The listing builds one solid part. Answer for the finished solid, in the listing's coordinates (mm). Round coordinates to 2 decimals unless told otherwise and drop trailing zeros. Write each loop counter-clockwise with the first axis right and the second up, starting at its lowest first coordinate (ties: lowest second). Pieces come first, ordered by that corner, then holes. Notation, with made-up numbers: (11.5, -38.5) - (49.5, -38.5) arc R6 cw to (49.5, -28.5) - close; hole circle Ø5 at (55.5, -10). An arc over 180 degrees is marked (long way). Use a Markdown table: item, result. Add a question column.
1) Find the intervals of material crossed by probe 1 along Z at (x, y) = (3.75, 444.5); probe 2 along Z at (x, y) = (1.25, 651); probe 3 along Y at (x, z) = (3.5, -644.5), in increasing order. Write a range as from..to.
2) A cutting plane is placed at A-A (x = 3). Give the vertices of the cut face in (y, z) (3 decimals), then the cut area to 3 significant figures.
3) A cutting plane is placed at B-B (z = -222). Give the vertices of the cut face in (x, y).
4) This flat-tipped pin is pushed along its axis until it touches: P1, Ø1.9, axis at x = 4.5, z = -584, coming from the +Y side. Where does it stop, or does it pass through?
```python
from build123d import *

# Parameters (mm, degrees)
SKETCH1_R           = 2.45745
BOSS_EXTRUDE1_DEPTH = 6.35


with BuildPart() as part:
    # Sketch1 → Boss-Extrude1 (new body)
    with BuildSketch(Plane(origin=(0, 0, 0), x_dir=(0, 0, -1), z_dir=(1, 0, 0))):
        with BuildLine():
            Line((457.2, 546.1), (755.65, 546.1))
            ThreePointArc((755.65, 546.1), (760.140128061, 544.240128061), (762, 539.75))
            Line((762, 539.75), (762, 6.35))
            ThreePointArc((762, 6.35), (760.140128061, 1.859871939), (755.65, 0))
            Line((755.65, 0), (6.35, 0))
            ThreePointArc((6.35, 0), (1.859871939, 1.859871939), (0, 6.35))
            Line((0, 6.35), (0, 539.75))
            ThreePointArc((0, 539.75), (1.859871939, 544.240128061), (6.35, 546.1))
            Line((6.35, 546.1), (304.8, 546.1))
            ThreePointArc((304.8, 546.1), (313.780256121, 549.819743879), (317.5, 558.8))
            Line((317.5, 558.8), (317.5, 685.8))
            ThreePointArc((317.5, 685.8), (321.219743879, 694.780256121), (330.2, 698.5))
            Line((330.2, 698.5), (431.8, 698.5))
            ThreePointArc((431.8, 698.5), (440.780256121, 694.780256121), (444.5, 685.8))
            Line((444.5, 685.8), (444.5, 558.8))
            ThreePointArc((444.5, 558.8), (448.219743879, 549.819743879), (457.2, 546.1))
        make_face()
        with Locations((53.975, 444.5)):
            Circle(SKETCH1_R, mode=Mode.SUBTRACT)
        with Locations((708.025, 444.5)):
            Circle(SKETCH1_R, mode=Mode.SUBTRACT)
        with Locations((708.025, 238.125)):
            Circle(SKETCH1_R, mode=Mode.SUBTRACT)
        with Locations((53.975, 238.125)):
            Circle(SKETCH1_R, mode=Mode.SUBTRACT)
        with Locations((53.975, 187.325)):
            Circle(SKETCH1_R, mode=Mode.SUBTRACT)
        with Locations((708.025, 187.325)):
            Circle(SKETCH1_R, mode=Mode.SUBTRACT)
    extrude(amount=BOSS_EXTRUDE1_DEPTH)


solid = part.part
```
Entries:
| question | item | result |
|---|---|---|
| 1 | probe 1 | z = -762..-710.48, -705.57..-56.43, -51.52..0 |
| 1 | probe 2 | z = -444.5..-317.5 |
| 1 | probe 3 | y = 0..546.1 |
| 2 | outline | (0, -755.65) arc R6.35 ccw to (6.35, -762) - (539.75, -762) arc R6.35 ccw to (546.1, -755.65) - (546.1, -457.2) arc R12.7 cw to (558.8, -444.5) - (685.8, -444.5) arc R12.7 ccw to (698.5, -431.8) - (698.5, -330.2) arc R12.7 ccw to (685.8, -317.5) - (558.8, -317.5) arc R12.7 cw to (546.1, -304.8) - (546.1, -6.35) arc R6.35 ccw to (539.75, 0) - (6.35, 0) arc R6.35 ccw to (0, -6.35) - close; hole circle Ø4.915 at (187.325, -708.025); hole circle Ø4.915 at (187.325, -53.975); hole circle Ø4.915 at (238.125, -708.025); hole circle Ø4.915 at (238.125, -53.975); hole circle Ø4.915 at (444.5, -708.025); hole circle Ø4.915 at (444.5, -53.975) |
| 2 | area | 435,000 mm² |
| 3 | outline | (0, 0) - (6.35, 0) - (6.35, 546.1) - (0, 546.1) - close |
| 4 | P1 | stops at y = 546.1 |
